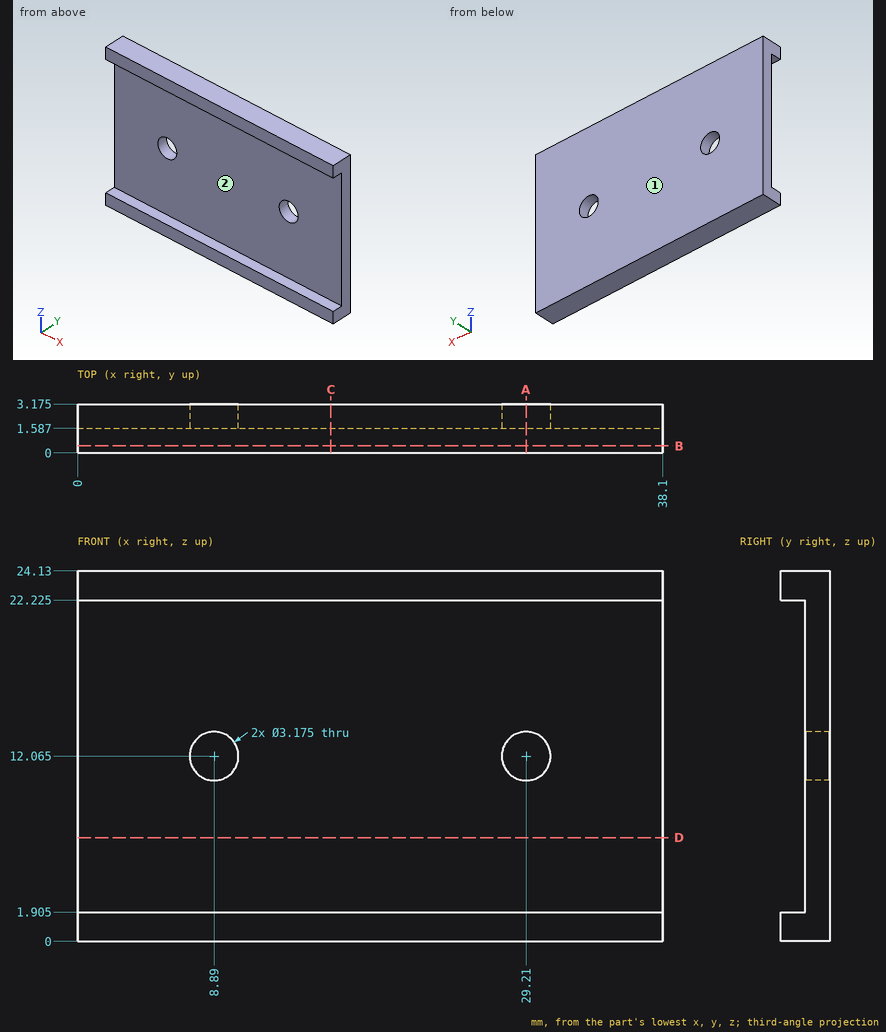
Geometry: see drawing. Coordinates: mm, zero at the bounding-box minimum. A direction names the side the tool comes from. Round coordinates to 2 decimals unless told otherwise and drop trailing zeros. Write each loop counter-clockwise with the first axis right and the second up, starting at its lowest first coordinate (ties: lowest second). Pieces come first, ordered by that corner, then holes. Notation, with made-up numbers: (45.5, -1.75) -> (59.5, -1.75) arc R22 ccw to (59.5, 26.25) -> close; hole circle Ø3 at (43.25, -22.75). An arc over 180 degrees is marked (long way). Answer as CSV lines item,"result".
1. Reachability of the marked faces 1 and 2 from +Z, -Z, +X, -X, +Y, -Y: full face, straight path, thin tool, end or side. Return the list, or none.
Geometry says:
face 1,"+Z, -Z, +X, -X, +Y"
face 2,"+X, -X, -Y"
2. Ray query, L1, parallel to Z at x = 8.89, y = 1.95; L2, parallel to Z at x = 20, y = 0.2 (1 decimal); L3, parallel to Y at x = 13, z = 22 (1 decimal). Return the intervals inside material, ascending. Write a range as [from, to].
Geometry says:
L1,"z = [0, 10.48], [13.65, 24.13]"
L2,"z = [0, 1.9], [22.2, 24.1]"
L3,"y = [1.6, 3.2]"
3. Section B-B (y = 0.45). Return the cut outline in (x, z) (1 decimal), plus the area to 3 significant figures.
Geometry says:
outline,"(0, 0) -> (38.1, 0) -> (38.1, 1.9) -> (0, 1.9) -> close; (0, 22.2) -> (38.1, 22.2) -> (38.1, 24.1) -> (0, 24.1) -> close"
area,"145 mm^2"
4. Section D-D (z = 6.75). Return the cut outline in (x, y) (1 decimal).
Geometry says:
outline,"(0, 1.6) -> (38.1, 1.6) -> (38.1, 3.2) -> (0, 3.2) -> close"
5. Section C-C (x = 16.5). Return the cut outline in (y, z) (1 decimal).
Geometry says:
outline,"(0, 0) -> (3.2, 0) -> (3.2, 24.1) -> (0, 24.1) -> (0, 22.2) -> (1.6, 22.2) -> (1.6, 1.9) -> (0, 1.9) -> close"
6. Contact query for flat-ended pins moving along their axis: P1, Ø2, axis at x = 6.5, z = 17.5, coming from the -Y side; P2, Ø3, axis at x = 8.89, z = 12.065, coming from the +Y side. Output: stop coordinate, or through.
Geometry says:
P1,"stops at y = 1.59"
P2,"passes through"
7. Section A-A (x = 29.21). Return the cut outline in (y, z) (1 decimal).
Geometry says:
outline,"(0, 0) -> (3.2, 0) -> (3.2, 10.5) -> (1.6, 10.5) -> (1.6, 1.9) -> (0, 1.9) -> close; (0, 22.2) -> (1.6, 22.2) -> (1.6, 13.7) -> (3.2, 13.7) -> (3.2, 24.1) -> (0, 24.1) -> close"
